from build123d import *

# Parameters (mm, degrees)
F1_DEPTH = 40
F2_R     = 2.625
F3_DEPTH = 25
F4_SIZE2 = 0.6999093082
F4_SIZE  = 8
F5_SIZE2 = 11.3425636392
F5_SIZE  = 2


with BuildPart() as f1:
    # F0 (on Top) → F1 (new body)
    with BuildSketch(Plane.XY):
        with BuildLine():
            ThreePointArc((0, 9), (-4.5, 4.5), (0, 0))
            Line((0, 0), (10, 0))
            ThreePointArc((10, 0), (14.5, 4.5), (10, 9))
            Line((10, 9), (0, 9))
        make_face()
    extrude(amount=F1_DEPTH)

    # F2 (on face) → F3 (cut)
    with BuildSketch(Plane.XZ):
        with Locations((5, 20)):
            Circle(F2_R)
    extrude(amount=-F3_DEPTH, mode=Mode.SUBTRACT)

    # F4
    f4_edges = [f1.edges().sort_by_distance(p)[0] for p in [
        (5, 0, 0),
        (14.5, 4.5, 0),
        (5, 9, 0),
        (-4.5, 4.5, 0),
    ]]
    chamfer(f4_edges, length=F4_SIZE, length2=F4_SIZE2)

    # F5
    f5_edges = [f1.edges().sort_by_distance(p)[0] for p in [
        (5, 0, 40),
        (14.5, 4.5, 40),
        (5, 9, 40),
        (-4.5, 4.5, 40),
    ]]
    f5_side = f1.faces().sort_by_distance((5, 4.5, 40))[0]
    chamfer(f5_edges, length=F5_SIZE, length2=F5_SIZE2, reference=f5_side)


solid = f1.part
Design review of the part built by this model. Coordinates are the model's own, in mm. Give positions to 0.01 mm unless a question says otherwise; leave off trailing zeros. Loops run counter-clockwise (first coordinate to the right, second up) from the corner with the lowest first, then second, coordinate; pieces in that order, holes last. Notation, with made-up numbers: M 30.25,-5.5 L 67.25,-5.5 A29 cw 67.25,28.5 Z; hole C 59.25,-38.5 d10. An arc over 180 degrees is marked long. Write item = value, one per line.
Q1. To check wall thickness, follow line 1 (Z direction, x = 5, y = 4) (3 decimals); line 2 (X direction, y = 4.75, z = 11); line 3 (Z direction, x = 7, y = 6.5). State the ranges of each line that lie inside material, in increasing order. Write a range as [from, to].
Output values:
line_1 = [0, 17.375], [22.625, 40]
line_2 = [-4.49, 14.49]
line_3 = [0, 18.3], [21.7, 40]
Q2. We need section D-D (x = 1.5). Give the boundary of the cut face in (y, z), plus the area to 3 significant figures.
Output values:
outline = M 0,8 L 0.7,0 L 8.3,0 L 9,8 L 9,28.66 L 7,40 L 2,40 L 0,28.66 Z
area = 332 mm^2
Q3. We need section C-C (z = 20). Give the boundary of the cut face in (x, y) (3 decimals).
Output values:
outline = M 0,0 L 2.375,0 L 2.375,9 L 0,9 A4.5 ccw Z; M 7.625,0 L 10,0 A4.5 ccw 10,9 L 7.625,9 Z
Q4. We need section B-B (x = 5). Give the boundary of the cut face in (y, z) (3 decimals).
Output values:
outline = M 0,8 L 0.7,0 L 8.3,0 L 9,8 L 9,17.375 L 0,17.375 Z; M 0,22.625 L 9,22.625 L 9,28.657 L 7,40 L 2,40 L 0,28.657 Z
Q5. We need section A-A (y = 4.5). Give the boundary of the cut face in (x, z) (3 decimals).
Output values:
outline = M -4.5,8 L -3.8,0 L 13.8,0 L 14.5,8 L 14.5,28.657 L 12.5,40 L -2.5,40 L -4.5,28.657 Z; hole C 5,20 d5.25
Q6. Insertion check: pin 1 (1 mm diameter, centred on x = 5, z = 30.5, fed in from -Y); pin 2 (3 mm diameter, centred on x = -2.5, z = 30.5, fed in from -Y). Each pin has a flat end and moves straight along its axis. Give the tip position at first contact, or say it passes through.
Output values:
pin_1 = 0.24
pin_2 = 0.36
Q7. Draft analysis for pull direction Y (two halves, no side actions). For faces 1 (the flat face through (4.93, 0.986, 34.249)), 2 (the flat face through (5.07, 8.014, 34.249)), 3 (the conical face through (13.513, 4.423, 34.249)), 4 (the flat face through (5, 5, 40)), state which applies: +Y half, -Y half, draft (parallel to the pull), parting line (faces both ways), or undercut.
Output values:
face_1 = -Y half
face_2 = +Y half
face_3 = parting line
face_4 = draft
